from build123d import *

# Parameters (mm, degrees)
F0_W     = 385
F0_H     = 205
F1_DEPTH = 15


with BuildPart() as f1:
    # F0 (on Front) → F1 (new body)
    with BuildSketch(Plane.XZ):
        with Locations((192.5, -102.5)):
            Rectangle(F0_W, F0_H)
        with BuildLine():
            ThreePointArc((43.81616, -35), (45.280627, -31.464466), (48.81616, -30))
            Line((48.81616, -30), (328.273739, -30))
            ThreePointArc((328.273739, -30), (331.809273, -31.464466), (333.273739, -35))
            Line((333.273739, -35), (333.273739, -120))
            ThreePointArc((333.273739, -120), (331.809273, -123.535534), (328.273739, -125))
            Line((328.273739, -125), (48.81616, -125))
            ThreePointArc((48.81616, -125), (45.280627, -123.535534), (43.81616, -120))
            Line((43.81616, -120), (43.81616, -35))
        make_face(mode=Mode.SUBTRACT)
    extrude(amount=F1_DEPTH)


solid = f1.part
Geometry check sheet. Reference: the model listing, model coordinates, mm. A direction names the side the tool comes from. Give positions to 0.01 mm unless a question says otherwise; leave off trailing zeros. Loops run counter-clockwise (first coordinate to the right, second up) from the corner with the lowest first, then second, coordinate; pieces in that order, holes last. Notation, with made-up numbers: M 50,41.25 L 98,41.25 A36 cw 98,78.25 Z; hole C -27.5,0 d11. An arc over 180 degrees is marked long. Write each question's results on one line, items separated by ' | '.
1) Section check C-C, the plane x = 161.5. Record the boundary of the cut face in (y, z).
Answers follow:
outline: M -15,-205 L 0,-205 L 0,-125 L -15,-125 Z; M -15,-30 L 0,-30 L 0,0 L -15,0 Z
2) Section check A-A, the plane y = -5.5. Record the boundary of the cut face in (x, z), plus the area to 3 significant figures.
Answers follow:
outline: M 0,-205 L 385,-205 L 385,0 L 0,0 Z; hole M 43.82,-120 A5 ccw 48.82,-125 L 328.27,-125 A5 ccw 333.27,-120 L 333.27,-35 A5 ccw 328.27,-30 L 48.82,-30 A5 ccw 43.82,-35 Z | area: 51,400 mm2
3) Release check for a two-part mould opening along Z. For faces 3 (the face through (191, -7, -125)), 4 (the face through (190, -7, 0)), 5 (the face through (190, -15, -147)) record: +Z half, -Z half, draft (parallel to the pull), parting line (faces both ways), or undercut.
Answers follow:
face 3: undercut | face 4: +Z half | face 5: draft
4) Gauge pin test, flat end, axial feed: pin 1 (2 mm diameter, centred on x = 147.5, y = -12.5, fed in from +Z). Record the tip position at first contact, or that the pin passes through.
Answers follow:
pin 1: z = 0
5) Section check B-B, the plane z = -100. Record the boundary of the cut face in (x, y), plus the area to 3 significant figures.
Answers follow:
outline: M 0,-15 L 43.82,-15 L 43.82,0 L 0,0 Z; M 333.27,-15 L 385,-15 L 385,0 L 333.27,0 Z | area: 1,430 mm2
6) Tool access check on faces 1 (the face through (43.816, -7, -78)), 2 (the face through (385, -7, -104)). Record the directions out of +Z, -Z, +X, -X, +Y, -Y that give a thin tool (end or side, any length) a straight path to the whole face; none if there is none.
Answers follow:
face 1: +Y, -Y | face 2: +Z, -Z, +X, +Y, -Y
7) Thickness scan on line 1 (Z direction, x = 299.5, y = -13.5); line 2 (X direction, y = -11, z = -76). Record the ranges inside material, lowest first.
Answers follow:
line 1: -205 to -125, -30 to 0 | line 2: 0 to 43.82, 333.27 to 385
